CAD build for the part. Positions are in the model's coordinates, mm. Face numbers are marked on the shaded views. A direction names the side the tool comes from. Round coordinates to 2 decimals unless told otherwise and drop trailing zeros. Order: outer loops, then holes, each group sorted by start corner. A loop starts at its lowest first (then second) coordinate and runs counter-clockwise, first axis right, second up. Notation, with made-up numbers: M 16,83.25 L 33,83.25 A11 ccw 33,101.25 Z; hole C 55.5,35.5 d7. An arc over 180 degrees is marked long. Answer as a JSON object with one key per item and string values.
```python
from build123d import *

# Parameters (mm, degrees)
SKETCH1_R           = 50.8
BOSS_EXTRUDE1_DEPTH = 12.7
SKETCH2_R           = 3.175
SKETCH2_R_2         = 2.38125
SKETCH2_R_3         = 1.5875
CUT_EXTRUDE1_DEPTH  = 73.955945611
FILLET1_R           = 2.54


with BuildPart() as part:
    # Sketch1 → Boss-Extrude1 (new body)
    with BuildSketch(Plane(origin=(0, 0, 0), x_dir=(1, 0, 0), z_dir=(0, 1, 0))):
        with Locations(Location((0, 0, 0), (0, 0, 270))):
            Circle(SKETCH1_R)
        with BuildLine():
            Line((-0.635, 2.295022127), (-0.635, 3.01625))
            Line((-0.635, 3.01625), (0.635, 3.01625))
            Line((0.635, 3.01625), (0.635, 2.295022127))
            ThreePointArc((0.635, 2.295022127), (0, -2.38125), (-0.635, 2.295022127))
        make_face(mode=Mode.SUBTRACT)
    extrude(amount=BOSS_EXTRUDE1_DEPTH)

    # Sketch2 → Cut-Extrude1 (cut, through all)
    with BuildSketch(Plane(origin=(0, 12.7, 0), x_dir=(1, 0, 0), z_dir=(0, 1, 0))):
        with BuildLine():
            Line((5.844661521, -11.275190983), (3.175, -41.789561795))
            ThreePointArc((3.175, -41.789561795), (36.295124673, -20.955), (37.778322127, 18.14515024))
            Line((37.778322127, 18.14515024), (12.686932584, 0.575970138))
            ThreePointArc((12.686932584, 0.575970138), (10.998522628, -6.35), (5.844661521, -11.275190983))
        make_face()
        with BuildLine():
            ThreePointArc((-37.778322127, 18.14515024), (-36.295124673, -20.955), (-3.175, -41.789561795))
            Line((-3.175, -41.789561795), (-5.844661521, -11.275190983))
            ThreePointArc((-5.844661521, -11.275190983), (-10.998522628, -6.35), (-12.686932584, 0.575970138))
            Line((-12.686932584, 0.575970138), (-37.778322127, 18.14515024))
        make_face()
        with BuildLine():
            ThreePointArc((34.603322127, 23.644411554), (0, 41.91), (-34.603322127, 23.644411554))
            Line((-34.603322127, 23.644411554), (-6.842271064, 10.699220845))
            ThreePointArc((-6.842271064, 10.699220845), (-3.564400038, 12.189546848), (0, 12.7))
            ThreePointArc((0, 12.7), (3.564400038, 12.189546848), (6.842271064, 10.699220845))
            Line((6.842271064, 10.699220845), (34.603322127, 23.644411554))
        make_face()
        with Locations(Location((0, -19.05, 0), (0, 0, 270))):
            Circle(SKETCH2_R)
        with Locations(Location((0, -27.94, 0), (0, 0, 270))):
            Circle(SKETCH2_R_2)
        with Locations(Location((0, -36.83, 0), (0, 0, 270))):
            Circle(SKETCH2_R_3)
        with Locations(Location((-16.497783942, 9.525, 0), (0, 0, 270))):
            Circle(SKETCH2_R)
        with Locations(Location((-24.196749782, 13.97, 0), (0, 0, 270))):
            Circle(SKETCH2_R_2)
        with Locations(Location((-31.895715621, 18.415, 0), (0, 0, 270))):
            Circle(SKETCH2_R_3)
        with Locations(Location((16.497783942, 9.525, 0), (0, 0, 270))):
            Circle(SKETCH2_R)
        with Locations(Location((24.196749782, 13.97, 0), (0, 0, 270))):
            Circle(SKETCH2_R_2)
        with Locations(Location((31.895715621, 18.415, 0), (0, 0, 270))):
            Circle(SKETCH2_R_3)
    extrude(amount=-CUT_EXTRUDE1_DEPTH, mode=Mode.SUBTRACT)

    # Fillet1
    fillet1_edges = [part.edges().sort_by_distance(p)[0] for p in [
        (-37.778322127, 6.35, -18.14515024),
        (-12.686932584, 6.35, -0.575970138),
        (-5.844661521, 6.35, 11.275190983),
        (-3.175, 6.35, 41.789561795),
        (3.175, 6.35, 41.789561795),
        (5.844661521, 6.35, 11.275190983),
        (12.686932584, 6.35, -0.575970138),
        (37.778322127, 6.35, -18.14515024),
        (-34.603322127, 6.35, -23.644411554),
        (34.603322127, 6.35, -23.644411554),
        (6.842271064, 6.35, -10.699220845),
        (-6.842271064, 6.35, -10.699220845),
    ]]
    fillet(fillet1_edges, radius=FILLET1_R)


solid = part.part
```
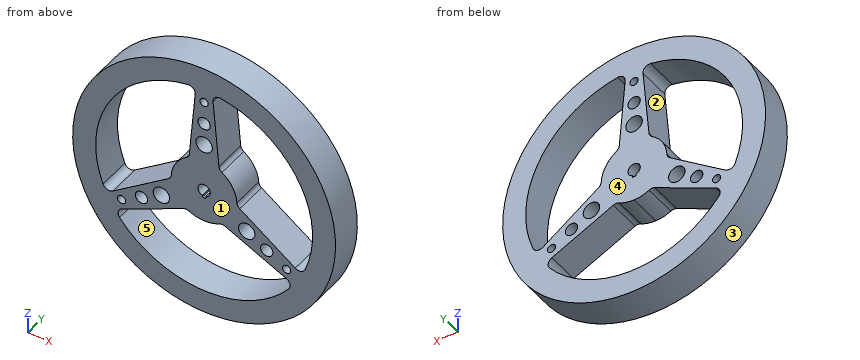
Item 1: Saw through at B-B on z = -36.5. List the corners of the cut face in (x, y), and give its area (3 significant figures).
Worked answers:
{"outline": "M -35.33,0 L -20.6,0 L -20.6,12.7 L -35.33,12.7 Z; M 20.6,0 L 35.33,0 L 35.33,12.7 L 20.6,12.7 Z", "area": "374 mm2"}
Item 2: Saw through at C-C on x = -29. List the corners of the cut face in (y, z), and give its area (3 significant figures).
Worked answers:
{"outline": "M 0,-41.71 L 12.7,-41.71 L 12.7,-30.26 L 0,-30.26 Z; M 0,-21.03 L 12.7,-21.03 L 12.7,-12 L 0,-12 Z; M 0,30.26 L 12.7,30.26 L 12.7,41.71 L 0,41.71 Z", "area": "406 mm2"}
Item 3: Saw through at D-D on z = 8.5. List the corners of the cut face in (x, y).
Worked answers:
{"outline": "M -50.08,0 L -41.04,0 L -41.04,12.7 L -50.08,12.7 Z; M -9.44,0 L 9.44,0 L 9.44,12.7 L -9.44,12.7 Z; M 41.04,0 L 50.08,0 L 50.08,12.7 L 41.04,12.7 Z"}
Item 4: Wall check: line 1 along X through (y, z) = (1.25, 20); line 2 along Z through (x, y) = (30.5, 11.25) (3 decimals); line 3 along X through (y, z) = (7, -1). Give the ranges that are in metal, low to high. Write a range as [from, to].
Worked answers:
{"line 1": "x = [-46.7, -36.83], [-5.08, -3.03], [3.03, 5.08], [36.83, 46.7]", "line 2": "z = [-40.625, -28.744], [-21.731, -19.171], [-17.659, -13.049], [28.744, 40.625]", "line 3": "x = [-50.79, -41.9], [-13.38, -2.16], [2.16, 13.38], [41.9, 50.79]"}
Item 5: Drop flat-ended pins along their axis: pin 1 Ø4 at (y, z) = (4.5, 9) entering from -X; pin 2 Ø1.5 at (y, z) = (4, -18.5) entering from +X; pin 3 Ø3 at (x, z) = (0, 36.83) entering from -Y; pin 4 Ø0.8 at (y, z) = (8, -2.5) entering from +X. Give the stop position or say it passes through.
Worked answers:
{"pin 1": "stops at x = -50.32", "pin 2": "stops at x = 47.6", "pin 3": "passes through", "pin 4": "stops at x = 50.76"}
Item 6: Two-plate mould, pull along Z, no slides. Class the marked faces 3, 4 and 5: released by +Z, released by -Z, zero draft, split by the parting line, or undercut.
Worked answers:
{"face 3": "split by the parting line", "face 4": "zero draft", "face 5": "undercut"}
Item 7: 3-axis set-ups, long thin cutter, end or side, ignore diameter. For the marked faces 1 and 2: which of +Z, -Z, +X, -X, +Y, -Y reach the whole face in a straight line?
Worked answers:
{"face 1": "+Z, -Z, +X, -X, -Y", "face 2": "+Y, -Y"}
Item 8: Saw through at A-A on z = 36.83. List the corners of the cut face in (x, y), and give its area (3 significant figures).
Worked answers:
{"outline": "M -34.99,0 L -20,0 L -20,12.7 L -34.99,12.7 Z; M -3.61,0 L -1.59,0 L -1.59,12.7 L -3.61,12.7 Z; M 1.59,0 L 3.61,0 L 3.61,12.7 L 1.59,12.7 Z; M 20,0 L 34.99,0 L 34.99,12.7 L 20,12.7 Z", "area": "432 mm2"}
